from build123d import *

# Parameters (mm, degrees)
F0_R         = 12.7
F1_DEPTH     = 25.4
F2_W         = 25.4
F2_H         = 12.7
F3_DEPTH     = 45.72
F4_R         = 5.08
F5_T1_DEPTH  = 15.24
F5_T6_DEPTH  = 53.34
F5_S7_R      = 12.7
F5_T8_DEPTH  = 28
F5_T10_ANGLE = 90
F5_T14_DEPTH = 53.34
F5_S15_R     = 12.7
F5_T16_DEPTH = 28
F5_T18_ANGLE = 90
F6_R         = 12.7
F7_DEPTH     = 25.4


# Not quite as in the source:
# - a fillet or chamfer that OpenCascade refuses, or shapes differently, is made with other operations: its cross-section is extruded or revolved along the edge and cut away or added


with BuildPart() as f1:
    # F0 (on Front) → F1 (new body, symmetric)
    with BuildSketch(Plane.XZ):
        Circle(F0_R)
    extrude(amount=F1_DEPTH, both=True)

    # F2 (on Top) → F3 (join)
    with BuildSketch(Plane.XY):
        with Locations((0, -19.05)):
            Rectangle(F2_W, F2_H)
    extrude(amount=F3_DEPTH)

    # F4
    f4_edges = [f1.edges().sort_by_distance(p)[0] for p in [
        (-12.7, -19.05, 45.72),
        (12.7, -19.05, 45.72),
        (0, -25.4, -12.7),
        (0, -25.4, 45.72),
    ]]
    fillet(f4_edges, radius=F4_R)

    # F5: fillet of radius 5.08 on 5 edges, made by hand

    # F5_s2 → F5_t1 (cut)
    with BuildSketch(Plane.YZ.offset(-7.62)):
        with BuildLine():
            ThreePointArc((-12.7, 40.64), (-14.1878975516, 44.2321024484), (-17.78, 45.72))
            Line((-17.78, 45.72), (-12.7, 45.72))
            Line((-12.7, 45.72), (-12.7, 40.64))
        make_face()
    extrude(amount=F5_T1_DEPTH, mode=Mode.SUBTRACT)


with BuildPart() as f5_tool4:
    # F5_s5 → F5_t6 (new body)
    with BuildSketch(Plane.XY.offset(-12.7)):
        with BuildLine():
            ThreePointArc((-12.7, -17.78), (-11.2121024484, -14.1878975516), (-7.62, -12.7))
            Line((-7.62, -12.7), (-12.7, -12.7))
            Line((-12.7, -12.7), (-12.7, -17.78))
        make_face()
    extrude(amount=F5_T6_DEPTH)

    # F5_s7 → F5_t8 (cut, symmetric)
    with BuildSketch(Plane.XZ.offset(15.2)):
        Circle(F5_S7_R)
    extrude(amount=F5_T8_DEPTH, both=True, mode=Mode.SUBTRACT)


with BuildPart() as f1_1:
    add(f1.part)

    # F5_t3: cut F5_tool4
    add(f5_tool4.part, mode=Mode.SUBTRACT)

    # F5_s9 → F5_t10 (revolve, cut)
    with BuildSketch(Plane.XY.offset(40.64)):
        with BuildLine():
            ThreePointArc((-7.62, -12.7), (-11.2121024484, -14.1878975516), (-12.7, -17.78))
            Line((-12.7, -17.78), (-12.7, -12.7))
            Line((-12.7, -12.7), (-7.62, -12.7))
        make_face()
    revolve(axis=Axis((-7.62, -12.7, 40.64), (0, 1, 0)), revolution_arc=F5_T10_ANGLE, mode=Mode.SUBTRACT)


with BuildPart() as f5_tool12:
    # F5_s13 → F5_t14 (new body)
    with BuildSketch(Plane.XY.offset(-12.7)):
        with BuildLine():
            ThreePointArc((7.62, -12.7), (11.2121024484, -14.1878975516), (12.7, -17.78))
            Line((12.7, -17.78), (12.7, -12.7))
            Line((12.7, -12.7), (7.62, -12.7))
        make_face()
    extrude(amount=F5_T14_DEPTH)

    # F5_s15 → F5_t16 (cut, symmetric)
    with BuildSketch(Plane.XZ.offset(15.2)):
        Circle(F5_S15_R)
    extrude(amount=F5_T16_DEPTH, both=True, mode=Mode.SUBTRACT)


with BuildPart() as f1_2:
    add(f1_1.part)

    # F5_t11: cut F5_tool12
    add(f5_tool12.part, mode=Mode.SUBTRACT)

    # F5_s17 → F5_t18 (revolve, cut)
    with BuildSketch(Plane.XY.offset(40.64)):
        with BuildLine():
            ThreePointArc((7.62, -12.7), (11.2121024484, -14.1878975516), (12.7, -17.78))
            Line((12.7, -17.78), (12.7, -12.7))
            Line((12.7, -12.7), (7.62, -12.7))
        make_face()
    revolve(axis=Axis((7.62, -12.7, 40.64), (0, -1, 0)), revolution_arc=F5_T18_ANGLE, mode=Mode.SUBTRACT)

    # F6 (on face) → F7 (join)
    with BuildSketch(Plane(origin=(0, 25.4, 0), x_dir=(-1, 0, 0), z_dir=(0, 1, 0))):
        Circle(F6_R)
    extrude(amount=F7_DEPTH)


solid = f1_2.part
Read the model definition and answer for the solid it produces. Units are mm, in the model's axes. A direction names the side the tool comes from. Coordinates: 2 decimals unless noted, no trailing zeros. Loops run counter-clockwise (first coordinate to the right, second up) from the corner with the lowest first, then second, coordinate; pieces in that order, holes last. Notation, with made-up numbers: (-17, -34.5) -> (31, -34.5) arc R27 ccw to (31, -15.5) -> close; hole circle Ø8 at (29.25, 83). An arc over 180 degrees is marked (long way). Answer in a Markdown table with one row per item.
Item 1: Straight lines are drawn through the part: line 1 along Y through (x, z) = (-1.5, 38.5); line 2 along X through (y, z) = (-17.5, 21.5); line 3 along X through (y, z) = (37.5, 10). For each, find the intervals that lie inside material, in ascending order. Write a range as [from, to].
Returned:
| item | result |
|---|---|
| line 1 | y = [-25.4, -12.7] |
| line 2 | x = [-12.69, 12.69] |
| line 3 | x = [-7.83, 7.83] |
Item 2: Each of these flat-tipped pins is pushed along its axis until it touches: P1, Ø3, axis at x = -1.5, z = 15, coming from the +Y side; P2, Ø6, axis at x = -6, y = 36, coming from the +Z side; P3, Ø5, axis at x = -8.5, z = 1.5, coming from the -Y side; P4, Ø1, axis at y = 41.5, z = 4.5, coming from the +X side. Where does it stop, or does it pass through?
Returned:
| item | result |
|---|---|
| P1 | stops at y = -12.7 |
| P2 | stops at z = 12.34 |
| P3 | stops at y = -25.4 |
| P4 | stops at x = 12.05 |
Item 3: A cutting plane is placed at A-A on x = 0. Determine the outline of the cut face in (y, z), plus the area to 3 significant figures.
Returned:
| item | result |
|---|---|
| outline | (-25.4, -7.62) arc R5.08 ccw to (-20.32, -12.7) -> (50.8, -12.7) -> (50.8, 12.7) -> (-12.7, 12.7) -> (-12.7, 40.64) arc R5.08 ccw to (-17.78, 45.72) -> (-20.32, 45.72) arc R5.08 ccw to (-25.4, 40.64) -> close |
| area | 2,340 mm^2 |
Item 4: For faces 1 (the cylindrical face through (-11.251, -14.228, 24.551)), 2 (the cylindrical face through (11.172, -14.149, 24.551)), 3 (the cylindrical face through (-11.251, -19.032, 44.192)), determine the directions among +Z, -Z, +X, -X, +Y, -Y from which every point of the face is accessible in a straight line to the end or side of a thin tool.
Returned:
| item | result |
|---|---|
| face 1 | +Z, -X, +Y |
| face 2 | +Z, +X, +Y |
| face 3 | +Z, -X, +Y, -Y |
Item 5: A cutting plane is placed at B-B on y = 42. Determine the outline of the cut face in (x, z), plus the area to 3 significant figures.
Returned:
| item | result |
|---|---|
| outline | circle Ø25.4 at (0, 0) |
| area | 507 mm^2 |
